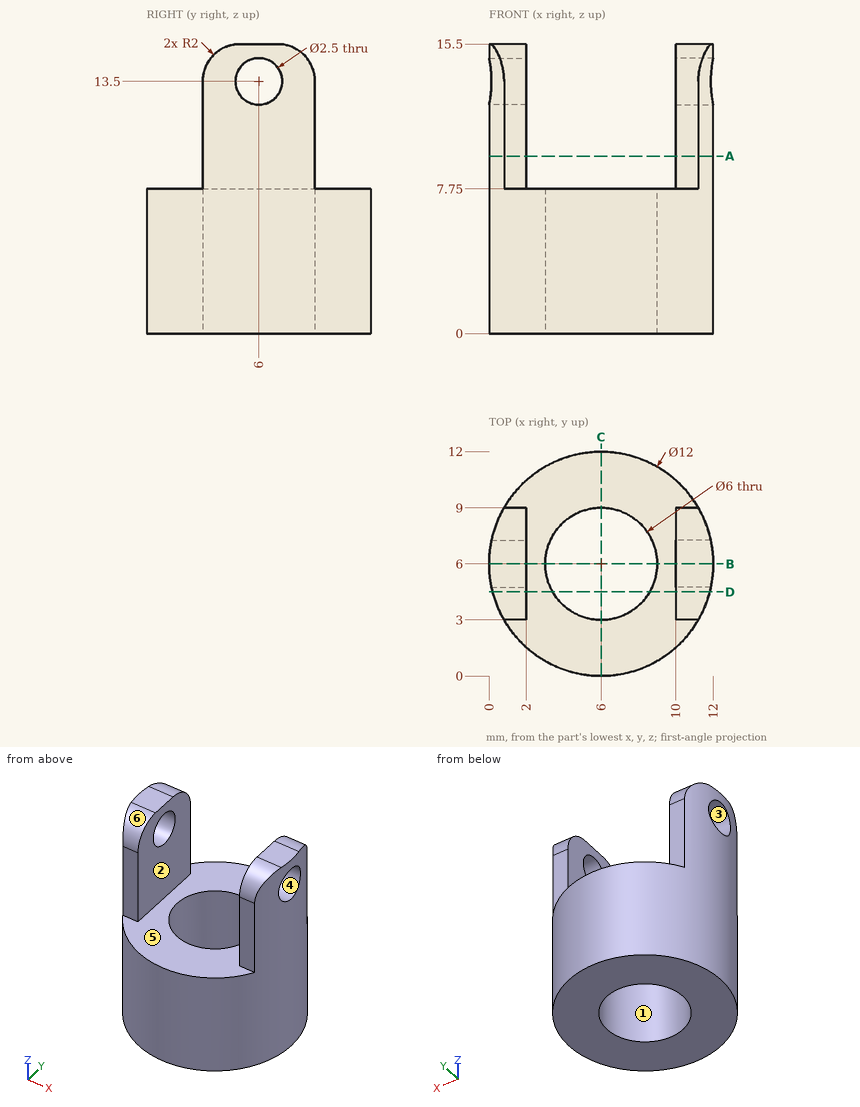
Study the drawing (mm; zero at the part's minimum x, y, z) and answer. A direction names the side the tool comes from. Coordinates: 2 decimals unless noted, no trailing zeros. Loops run counter-clockwise (first coordinate to the right, second up) from the corner with the lowest first, then second, coordinate; pieces in that order, holes last. Notation, with made-up numbers: M -38.5,37 L 17.5,37 A19 ccw 17.5,72 Z; hole C -18,75 d6. An arc over 180 degrees is marked long. Answer as a JSON object with one key per item and string values. Group by question number.
Item 1: Consider L1, parallel to Y at x = 6, z = 4; L2, parallel to X at y = 7, z = 1.5; L3, parallel to X at y = 4, z = 6. Determine where each line is inside the solid, lowest interval first.
Item 2: Determine the mould class of the marked faces 3, 4, 5 and 6 for opening direction Y: +Y half, -Y half, draft (parallel to the pull), parting line (faces both ways), or undercut.
Item 3: Which of the six approach directions +Z, -Z, +X, -X, +Y, -Y give full straight-line access (tool end or side, diameter ignored) to the marked faces 1 and 2?
Item 4: Section D-D (y = 4.5) is taken. Write down the section's boundary in (x, z).
Item 5: Each of these flat-tipped pins is pushed along its axis until it touches: P1, Ø4, axis at x = 9, z = 6, coming from the -Y side; P2, Ø3, axis at y = 4.5, z = 13.5, coming from the -X side; P3, Ø1.3, axis at x = 1.5, z = 10.5, coming from the -Y side. Where does it stop, or does it pass through?
Item 6: Section A-A (z = 9.5) is taken. Write down the section's boundary in (x, y), and give its area (3 significant figures).
Item 7: Section C-C (x = 6) is taken. Write down the section's boundary in (y, z).
Item 8: Section B-B (y = 6) is taken. Write down the section's boundary in (x, z).
Solved:
{
 "1": {"L1": "y = 0 to 3, 9 to 12", "L2": "x = 0.08 to 3.17, 8.83 to 11.92", "L3": "x = 0.34 to 3.76, 8.24 to 11.66"},
 "2": {"face 3": "undercut", "face 4": "undercut", "face 5": "draft", "face 6": "-Y half"},
 "3": {"face 1": "+Z, -Z", "face 2": "+Z, +Y, -Y"},
 "4": {"outline": "M 0.19,0 L 3.4,0 L 3.4,7.75 L 2,7.75 L 2,15.44 L 0.19,15.44 Z; M 8.6,0 L 11.81,0 L 11.81,15.44 L 10,15.44 L 10,7.75 L 8.6,7.75 Z"},
 "5": {"P1": "stops at y = 0.08", "P2": "stops at x = 0.02", "P3": "stops at y = 3"},
 "6": {"outline": "M 0.8,3 L 2,3 L 2,9 L 0.8,9 A6 ccw Z; M 10,3 L 11.2,3 A6 ccw 11.2,9 L 10,9 Z", "area": "20.9 mm2"},
 "7": {"outline": "M 0,0 L 3,0 L 3,7.75 L 0,7.75 Z; M 9,0 L 12,0 L 12,7.75 L 9,7.75 Z"},
 "8": {"outline": "M 0,0 L 3,0 L 3,7.75 L 2,7.75 L 2,12.25 L 0,12.25 Z; M 0,14.75 L 2,14.75 L 2,15.5 L 0,15.5 Z; M 9,0 L 12,0 L 12,12.25 L 10,12.25 L 10,7.75 L 9,7.75 Z; M 10,14.75 L 12,14.75 L 12,15.5 L 10,15.5 Z"}
}
